For this review, take the finished solid that the model builds, in its own axes (mm). A direction names the side the tool comes from. Round coordinates to 2 decimals unless told otherwise and drop trailing zeros. Order: outer loops, then holes, each group sorted by start corner. A loop starts at its lowest first (then second) coordinate and runs counter-clockwise, first axis right, second up.
```python
from build123d import *

# Parameters (mm, degrees)
BOSS_EXTRUDE1_DEPTH = 40
BOSS_EXTRUDE2_START = -10
SKETCH1_3_R         = 2
SKETCH1_3_R_2       = 1
BOSS_EXTRUDE2_DEPTH = 10
BOSS_EXTRUDE3_START = -30
SKETCH1_4_R         = 2
SKETCH1_4_R_2       = 1
BOSS_EXTRUDE3_DEPTH = 10
SKETCH2_R           = 2
CUT_EXTRUDE1_DEPTH  = 10
FILLET1_R           = 3
FILLET2_R           = 3


with BuildPart() as part:
    # Sketch1 → Boss-Extrude1 (new body)
    with BuildSketch(Plane.XY):
        with BuildLine():
            Line((33.441058941, -2), (33.441058941, 0))
            Line((33.441058941, 0), (13.441058941, 0))
            ThreePointArc((13.441058941, 0), (13.640859786, -0.48236191), (13.709008133, -1))
            ThreePointArc((13.709008133, -1), (13.640859786, -1.51763809), (13.441058941, -2))
            Line((13.441058941, -2), (33.441058941, -2))
        make_face()
    extrude(amount=-BOSS_EXTRUDE1_DEPTH)

    # Sketch1_3 → Boss-Extrude2 (add)
    with BuildSketch(Plane.XY.offset(BOSS_EXTRUDE2_START)):
        with Locations((11.709008133, -1)):
            Circle(SKETCH1_3_R)
        with Locations((11.709008133, -1)):
            Circle(SKETCH1_3_R_2, mode=Mode.SUBTRACT)
    extrude(amount=-BOSS_EXTRUDE2_DEPTH)

    # Sketch1_4 → Boss-Extrude3 (add)
    with BuildSketch(Plane.XY.offset(BOSS_EXTRUDE3_START)):
        with Locations((11.709008133, -1)):
            Circle(SKETCH1_4_R)
        with Locations((11.709008133, -1)):
            Circle(SKETCH1_4_R_2, mode=Mode.SUBTRACT)
    extrude(amount=-BOSS_EXTRUDE3_DEPTH)

    # Sketch2 → Cut-Extrude1 (cut)
    with BuildSketch(Plane(origin=(0, 0, 0), x_dir=(1, 0, 0), z_dir=(0, 1, 0))):
        with Locations((18.441058941, 30)):
            Circle(SKETCH2_R)
        with Locations((18.441058941, 10)):
            Circle(SKETCH2_R)
        with Locations((28.441058941, 20)):
            Circle(SKETCH2_R)
    extrude(amount=-CUT_EXTRUDE1_DEPTH, mode=Mode.SUBTRACT)

    # Fillet1
    fillet1_edges = [part.edges().sort_by_distance(p)[0] for p in [
        (33.441058941, -1, 0),
    ]]
    fillet(fillet1_edges, radius=FILLET1_R)

    # Fillet2
    fillet2_edges = [part.edges().sort_by_distance(p)[0] for p in [
        (33.441058941, -1, -40),
    ]]
    fillet(fillet2_edges, radius=FILLET2_R)


solid = part.part
```
Q1. Take a section at A-A, the plane z = -14.5. State the section outline as (x, y) points, plus the area to 3 significant figures.
Q2. Wall thickness on line 1 (X direction, y = -1.7, z = -10.5); line 2 (Y direction, x = 14.5, z = -28.5); line 3 (X direction, y = -1.1, z = -31.5): over which ranges is each line inside the solid? List them lowest first.
Q3. Take a section at C-C, the plane y = -1.4. State the section outline as (x, z) points, plus the area to 3 significant figures.
Q4. Tool access review of faces 5 (the face through (23, -2, -20)), 6 (the face through (10.71, -0.96, -34.93)), 7 (the face through (24, 0, -20)): name each direction out of +Z, -Z, +X, -X, +Y, -Y from which nothing blocks a thin tool from reaching the whole face with its end or side.
Q5. Mouldability with a two-part tool opening along Z and no side actions: class faces 1 (the face through (20, -1, -40)), 2 (the face through (18.007, -0.986, -28.048)), 3 (the face through (18.181, -0.986, -11.983)), 4 (the face through (9.71, -0.93, -14.93)) as +Z half, -Z half, draft (parallel to the pull), parting line (faces both ways), or undercut.
Q6. Take a section at B-B, the plane x = 19.5. State the section outline as (y, z) points.
Q7. Take a section at D-D, the plane x = 27.5. State the section outline as (y, z) points, plus the area to 3 significant figures.
Q8. Clearance check with flat-ended pins moving along their axes: pin 1 (4.5 mm diameter, centred on x = 28.44, z = -20, fed in from -Y); pin 2 (10 mm diameter, centred on x = 24.5, z = -19, fed in from +Y); pin 3 (1.2 mm diameter, centred on x = 11, y = -2, fed in from +Z). State where each tip first meets the part, or that it passes through.
Working result:
1. outline: (13.44, -2) - (33.44, -2) - (33.44, 0) - (13.44, 0) arc R2 ccw (long way) to start; hole circle Ø2 at (11.71, -1)
1. area: 49.1 mm2
2. line 1: x = 9.84 to 10.99, 12.42 to 16.5, 20.38 to 33.44
2. line 2: y = -2 to 0
2. line 3: x = 9.71 to 10.71, 12.7 to 17.12, 19.76 to 33.44
3. outline: (9.75, -40) - (10.79, -40) - (10.79, -30) - (9.75, -30) - close; (9.75, -20) - (10.79, -20) - (10.79, -10) - (9.75, -10) - close; (12.63, -40) - (30.44, -40) arc R3 ccw to (33.44, -37) - (33.44, -3) arc R3 ccw to (30.44, 0) - (13.67, 0) - (13.67, -10) - (12.63, -10) - (12.63, -20) - (13.67, -20) - (13.67, -30) - (12.63, -30) - close; hole circle Ø4 at (18.44, -30); hole circle Ø4 at (18.44, -10); hole circle Ø4 at (28.44, -20)
3. area: 791 mm2
4. face 5: +Z, -Z, +X, -Y
4. face 6: +Z, -Z
4. face 7: +Z, -Z, +X, +Y
5. face 1: -Z half
5. face 2: undercut
5. face 3: undercut
5. face 4: draft
6. outline: (-2, -40) - (0, -40) - (0, -31.7) - (-2, -31.7) - close; (-2, -28.3) - (0, -28.3) - (0, -11.7) - (-2, -11.7) - close; (-2, -8.3) - (0, -8.3) - (0, 0) - (-2, 0) - close
7. outline: (-2, -40) - (0, -40) - (0, -21.76) - (-2, -21.76) - close; (-2, -18.24) - (0, -18.24) - (0, 0) - (-2, 0) - close
7. area: 72.9 mm2
8. pin 1: stops at y = -2
8. pin 2: stops at y = 0
8. pin 3: stops at z = -10
